Input: part model. Units: mm. Frame: model coordinates. Face numbers are marked on the shaded views. A direction names the side the tool comes from. Coordinates: 2 decimals unless noted, no trailing zeros. Order: outer loops, then holes, each group sorted by start corner. A loop starts at its lowest first (then second) coordinate and runs counter-clockwise, first axis right, second up. Notation, with made-up numbers: (48.5, -13.5) -> (99.5, -13.5) arc R22 ccw to (99.5, 0.5) -> close; hole circle Ø9 at (-33, 1). An arc over 180 degrees is marked (long way). One line per question, with ' | ' between items.
```python
from build123d import *

# Parameters (mm, degrees)
F2_DEPTH = 25.4
F3_D     = 9.525


with BuildPart() as f2:
    # F1 (on Top) → F2 (new body)
    with BuildSketch(Plane.XY):
        with BuildLine():
            ThreePointArc((7.9375, 0), (5.6126600757, 5.6126600757), (0, 7.9375))
            ThreePointArc((0, 7.9375), (-7.9375, 0), (0, -7.9375))
            ThreePointArc((0, -7.9375), (5.6126600757, -5.6126600757), (7.9375, 0))
        make_face()
        with BuildLine():
            ThreePointArc((-144.0602539291, -68.2625), (-165.5292616255, -63.5029355815), (-182.9753116396, -50.1161105721))
            Line((-182.9753116396, -50.1161105721), (-268.4978463522, 51.8056774194))
            ThreePointArc((-268.4978463522, 51.8056774194), (-279.6804507713, 52.7840285348), (-280.6588018867, 41.6014241157))
            Line((-280.6588018867, 41.6014241157), (-195.1362671741, -60.3203638759))
            ThreePointArc((-195.1362671741, -60.3203638759), (-172.2383265307, -77.8905717007), (-144.0602539291, -84.1375))
            Line((-144.0602539291, -84.1375), (-71.4375, -84.1375))
            ThreePointArc((-71.4375, -84.1375), (-51.2319237276, -75.7680762724), (-42.8625, -55.5625))
            Line((-42.8625, -55.5625), (-42.8625, -20.6375))
            ThreePointArc((-42.8625, -20.6375), (-39.1427561211, -11.6572438789), (-30.1625, -7.9375))
            Line((-30.1625, -7.9375), (0, -7.9375))
            ThreePointArc((0, -7.9375), (-7.9375, 0), (0, 7.9375))
            Line((0, 7.9375), (-52.3875, 7.9375))
            ThreePointArc((-52.3875, 7.9375), (-56.8776280605, 6.0776280605), (-58.7375, 1.5875))
            Line((-58.7375, 1.5875), (-58.7375, -55.5625))
            ThreePointArc((-58.7375, -55.5625), (-62.4572438789, -64.5427561211), (-71.4375, -68.2625))
            Line((-71.4375, -68.2625), (-144.0602539291, -68.2625))
        make_face()
    extrude(amount=F2_DEPTH)

    # F3 (through all)
    with Locations(Plane(origin=(0, 0, 0), x_dir=(1, 0, 0), z_dir=(0, 0, -1))):
        with Locations((-274.5783241194, -46.7035507676), (0, 0), (-50.8, 0)):
            Hole(F3_D / 2)


solid = f2.part
```
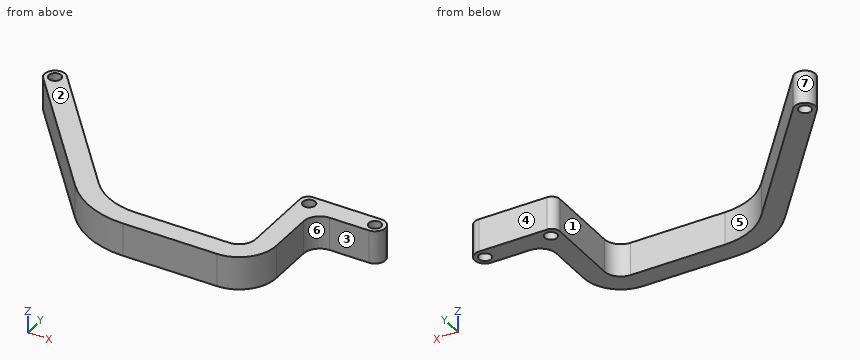
1. Cut plane C-C, the plane x = -250. Return loops of the section in (y, z).
Recorded:
outline: (5.06, 0) -> (29.76, 0) -> (29.76, 25.4) -> (5.06, 25.4) -> close
2. Cut plane A-A, the plane y = -17.5. Return loops of the section in (x, z).
Recorded:
outline: (-231.07, 0) -> (-210.34, 0) -> (-210.34, 25.4) -> (-231.07, 25.4) -> close; (-58.74, 0) -> (-42.47, 0) -> (-42.47, 25.4) -> (-58.74, 25.4) -> close
3. Pin query (flat end, axial travel): pin 1 Ø12.5 at (y, z) = (-30.5, 16.5) entering from +X; pin 2 Ø12 at (y, z) = (14, 7.5) entering from +X; pin 3 Ø2 at (x, z) = (-51, 19) entering from -Y. Return the tip coordinate at first contact, or that it passes through.
Recorded:
pin 1: stops at x = -42.86 | pin 2: stops at x = -231.74 | pin 3: stops at y = -76.51
4. Cut plane B-B, the plane z = 18.5. State how many separate pieces and enclosed holes the cut face has, and give its area (3 significant figures).
Recorded:
separate pieces: 1 | enclosed holes: 3 | area: 6,290 mm^2
5. Cut plane D-D, the plane y = 37. Return loops of the section in (x, z), and give its area (3 significant figures).
Recorded:
outline: (-276.8, 0) -> (-256.07, 0) -> (-256.07, 25.4) -> (-276.8, 25.4) -> close | area: 526 mm^2
6. Mould query, pull axis X, two halves, no side actions, for the marked faces 4, 5, 6 and 7. Classes: released by +X, released by -X, zero draft, split by the parting line, or undercut.
Recorded:
face 4: zero draft | face 5: undercut | face 6: released by +X | face 7: split by the parting line
7. Ray query, line 1 (Y direction, x = 0, z = 20); line 2 (X direction, y = 3, z = 16.25); line 3 (X direction, y = -23, z = 16). Return the intervals inside material, ascending. Write a range as [from, to].
Recorded:
line 1: y = [-7.94, -4.76], [4.76, 7.94] | line 2: x = [-248.27, -227.55], [-58.58, -54.5], [-47.1, -3.7], [3.7, 7.35] | line 3: x = [-226.45, -205.73], [-58.74, -42.86]
8. Access query for the marked faces 1, 2 and 3. Directions: +Z, -Z, +X, -X, +Y, -Y. A direction counts if a zero-diameter tool reaches every point of the face in a straight line with its end or side. Return the directions, or none.
Recorded:
face 1: +Z, -Z, +Y | face 2: +Z, +X, -X, +Y, -Y | face 3: +Z, -Z, +X, -Y
